CAD build for the part. Positions are in the model's coordinates, mm. A direction names the side the tool comes from. Coordinates: 2 decimals unless noted, no trailing zeros. Loops run counter-clockwise (first coordinate to the right, second up) from the corner with the lowest first, then second, coordinate; pieces in that order, holes last. Notation, with made-up numbers: (78, 55.25) -> (135, 55.25) arc R12 cw to (135, 62.25) -> close; hole circle Ø7 at (40, -25). An arc over 180 degrees is marked (long way). Write each question's results on one line, items separated by ' | '.
Autodesk Inventor part; units mm, degrees
ref_plane "YZ Plane" through (0, 0, 0) normal (1, 0, 0) x (0, 1, 0)
ref_plane "XZ Plane" through (0, 0, 0) normal (0, 1, 0) x (-1, 0, 0)
ref_plane "XY Plane" through (0, 0, 0) normal (0, 0, 1) x (1, 0, 0)
sketch "Sketch1" plane through (0, 0, 0) normal (0, 0, 1) x (1, 0, 0)
  circle A0 centre (0, 0) radius 3
  circle A1 centre (0, 0) radius 4.5
  line L0 (0, 0) -> (7.62, 0) construction
  line L1 (0, 0) -> (-7.62, 0) construction
  line L2 (10, -4.5) -> (-10, -4.5)
  line L3 (-10, -4.5) -> (-10, 4.5)
  line L4 (-10, 4.5) -> (10, 4.5)
  line L5 (10, 4.5) -> (10, -4.5)
  line L6 (10, -4.5) -> (-10, 4.5) construction
  line L7 (-10, -4.5) -> (10, 4.5) construction
  circle A2 centre (0, 0) radius 1.5
  dimension "d0" = 6
  dimension "d1" = 9
  dimension "d2" = 7.62
  dimension "d3" = 7.62
  dimension "d4" = 20
  dimension "d5" = 9
  dimension "d8" = 3
extrude "Extrusion1" add sketch "Sketch1" against normal blind 2 contours A1 | A1 L4 L5 L2 | A1 L2 L3 L4
extrude "Extrusion2" add sketch "Sketch1" along normal blind 1 contours A0 | A1
extrude "Extrusion3" add sketch "Sketch1" along normal blind 4 contours A1
hole "Hole1" at (-7.62, 0, 0) at (7.62, 0, 0) direction (0, 0, -1) diameter 2 end through all
properties part number "orczyk"
1) Two-plate mould, pull along Y, no slides. Class faces 1 (the flat face through (0, 4.5, -1)), 2 (the flat face through (0, -4.5, -1)), 3 (the cylindrical face through (6.63, 0.13, -1.01)): pulls with the +Y half, pulls with the -Y half, needs draft (parallel to the pull), parting line crosses it, or undercut.
Outcome:
face 1: pulls with the +Y half | face 2: pulls with the -Y half | face 3: undercut
2) Slice it at D-D (x = -2). Write the cut outline in (y, z).
Outcome:
outline: (-4.5, -2) -> (-2.24, -2) -> (-2.24, 0) -> (2.24, 0) -> (2.24, -2) -> (4.5, -2) -> (4.5, 0) -> (4.03, 0) -> (4.03, 4) -> (2.24, 4) -> (2.24, 1) -> (-2.24, 1) -> (-2.24, 4) -> (-4.03, 4) -> (-4.03, 0) -> (-4.5, 0) -> close
3) Slice it at A-A (x = -7.62). Write the cut outline in (y, z), then the cut area to 3 significant figures.
Outcome:
outline: (-4.5, -2) -> (-1, -2) -> (-1, 0) -> (-4.5, 0) -> close; (1, -2) -> (4.5, -2) -> (4.5, 0) -> (1, 0) -> close | area: 14.0 mm^2
4) Which spindle directions (+Z, -Z, +X, -X, +Y, -Y) get a long thin tool onto all of the face, cutting with end or side? Do faces 4 (the cylindrical face through (-0.59, -4.46, 1.97)), 5 (the cylindrical face through (-8.61, 0.13, -1.01)), 6 (the flat face through (1.3, -1.3, 0)). Say none if no direction does.
Outcome:
face 4: +Z | face 5: +Z, -Z | face 6: -Z
5) Slice it at C-C (y = 0). Write the cut outline in (x, z).
Outcome:
outline: (-10, -2) -> (-8.62, -2) -> (-8.62, 0) -> (-10, 0) -> close; (-6.62, -2) -> (-3, -2) -> (-3, 0) -> (-1.5, 0) -> (-1.5, 1) -> (-3, 1) -> (-3, 4) -> (-4.5, 4) -> (-4.5, 0) -> (-6.62, 0) -> close; (1.5, 0) -> (3, 0) -> (3, -2) -> (6.62, -2) -> (6.62, 0) -> (4.5, 0) -> (4.5, 4) -> (3, 4) -> (3, 1) -> (1.5, 1) -> close; (8.62, -2) -> (10, -2) -> (10, 0) -> (8.62, 0) -> close
6) Slice it at B-B (z = -1). Write the cut outline in (x, y), then the cut area to 3 significant figures.
Outcome:
outline: (-10, -4.5) -> (10, -4.5) -> (10, 4.5) -> (-10, 4.5) -> close; hole circle Ø2 at (-7.62, 0); hole circle Ø6 at (0, 0); hole circle Ø2 at (7.62, 0) | area: 145 mm^2
7) Pin check, flat tips, straight feed: pin 1 (3 mm diameter, centred on x = 0, y = 0.5, fed in from -Z); pin 2 (2.5 mm diameter, centred on x = 7.62, y = 0, fed in from +Z); pin 3 (1.8 mm diameter, centred on x = 0, y = -1, fed in from +Z). Stop position of each tip, or through.
Outcome:
pin 1: stops at z = 0 | pin 2: stops at z = 0 | pin 3: stops at z = 1
8) Drill centre lines: L1, parallel to Y at x = 0, z = -0.8; L2, parallel to Y at x = -7.62, z = -0.75. Where is each one in solid material? Low to high. Write a range as from..to.
Outcome:
L1: y = -4.5..-3, 3..4.5 | L2: y = -4.5..-1, 1..4.5
